CAD build for the part. Positions are in the model's coordinates, mm. A direction names the side the tool comes from. Round coordinates to 2 decimals unless told otherwise and drop trailing zeros. Loops run counter-clockwise (first coordinate to the right, second up) from the corner with the lowest first, then second, coordinate; pieces in that order, holes last. Notation, with made-up numbers: M 75,69 L 79,69 A15 ccw 79,92 Z; hole C 30.25,26 d2. An arc over 180 degrees is marked long. Use one line per item in the form item = value.
from build123d import *

# Parameters (mm, degrees)
SKETCH3_R           = 26.5
BOSS_EXTRUDE1_DEPTH = 37
SKETCH4_OUTSIDE_W   = 71.718
SKETCH4_OUTSIDE_H   = 71.718
SKETCH4_OUTSIDE_R   = 18.5
CUT_EXTRUDE1_DEPTH  = 1
SKETCH5_R           = 7.5
CUT_EXTRUDE2_DEPTH  = 2
CUT_EXTRUDE3_START  = -24.5
SKETCH6_W           = 30
SKETCH6_H           = 10
CUT_EXTRUDE3_DEPTH  = 29.16402947
CIRPATTERN1_COUNT   = 3
CIRPATTERN2_COUNT   = 3
CIRPATTERN3_COUNT   = 6


with BuildPart() as part:
    # Sketch3 → Boss-Extrude1 (new body)
    with BuildSketch(Plane.XY):
        Circle(SKETCH3_R)
    extrude(amount=-BOSS_EXTRUDE1_DEPTH)

    # Sketch4 outside → Cut-Extrude1 (cut)
    with BuildSketch(Plane.XY):
        Rectangle(SKETCH4_OUTSIDE_W, SKETCH4_OUTSIDE_H)
        Circle(SKETCH4_OUTSIDE_R, mode=Mode.SUBTRACT)
    extrude(amount=-CUT_EXTRUDE1_DEPTH, mode=Mode.SUBTRACT)

    # Sketch5 → Cut-Extrude2 (cut)
    with BuildSketch(Plane.XY):
        Circle(SKETCH5_R)
    extrude(amount=-CUT_EXTRUDE2_DEPTH, mode=Mode.SUBTRACT)

    # Sketch6 → Cut-Extrude3 (cut, through all)
    with BuildSketch(Plane.XY.offset(CUT_EXTRUDE3_START)):
        with Locations((0, -28)):
            Rectangle(SKETCH6_W, SKETCH6_H)
    extrude(amount=-CUT_EXTRUDE3_DEPTH, mode=Mode.SUBTRACT)

    # Sketch8 → M2.5x0.45 Tapped Hole1 (revolve, cut)
    with BuildSketch(Plane(origin=(-5.878275914, -23.011048917, -1), x_dir=(0, -1, 0), z_dir=(1, 0, 0))):
        Polygon((0, 0), (0, 6.965882135), (1.025, 6.35), (1.025, 0), align=None)
    m2_5x0_45_tapped_hole1 = revolve(axis=Axis((-5.878275914, -23.011048917, 5.35), (0, 0, -1)), mode=Mode.SUBTRACT)

    # Sketch10 → M2.5x0.45 Tapped Hole2 (revolve, cut)
    with BuildSketch(Plane(origin=(4.059528293, 12.875178835, 0), x_dir=(0, -1, 0), z_dir=(1, 0, 0))):
        Polygon((0, 0), (0, 4.965882135), (1.025, 4.35), (1.025, 0), align=None)
    m2_5x0_45_tapped_hole2 = revolve(axis=Axis((4.059528293, 12.875178835, 6.35), (0, 0, -1)), mode=Mode.SUBTRACT)

    # Sketch12 → M2.5x0.45 Tapped Hole3 (revolve, cut)
    with BuildSketch(Plane(origin=(0, 22.5, -37), x_dir=(0, 1, 0), z_dir=(1, 0, 0))):
        Polygon((0, 0), (0, 6.965882135), (1.025, 6.35), (1.025, 0), align=None)
    m2_5x0_45_tapped_hole3 = revolve(axis=Axis((0, 22.5, -43.35), (0, 0, 1)), mode=Mode.SUBTRACT)

    # CirPattern1: M2.5x0.45 Tapped Hole1 ×3 about axis
    cirpattern1_axis = Axis((0, 0, 0), (0, 0, 1))
    for i in range(1, CIRPATTERN1_COUNT):
        add(m2_5x0_45_tapped_hole1.rotate(cirpattern1_axis, i * 360 / CIRPATTERN1_COUNT), mode=Mode.SUBTRACT)

    # CirPattern2: M2.5x0.45 Tapped Hole2 ×3 about axis
    cirpattern2_axis = Axis((0, 0, 0), (0, 0, 1))
    for i in range(1, CIRPATTERN2_COUNT):
        add(m2_5x0_45_tapped_hole2.rotate(cirpattern2_axis, i * 360 / CIRPATTERN2_COUNT), mode=Mode.SUBTRACT)

    # CirPattern3: M2.5x0.45 Tapped Hole3 ×6 about axis, 1 skipped
    cirpattern3_axis = Axis((0, 0, 0), (0, 0, -1))
    add([m2_5x0_45_tapped_hole3.rotate(cirpattern3_axis, i * 360 / CIRPATTERN3_COUNT) for i in range(1, CIRPATTERN3_COUNT) if i not in (3,)], mode=Mode.SUBTRACT)


solid = part.part
1. Cut at D-D on z = -25.5. Write the cut outline in (x, y), and give its area (3 significant figures).
Completed:
outline = M -13.16,-23 L 13.16,-23 A26.5 ccw long Z
area = 2,140 mm2
2. Cut at A-A on y = 0. Write the cut outline in (x, z).
Completed:
outline = M -26.5,-37 L 26.5,-37 L 26.5,-1 L 18.5,-1 L 18.5,0 L 7.5,0 L 7.5,-2 L -7.5,-2 L -7.5,0 L -18.5,0 L -18.5,-1 L -26.5,-1 Z
3. Cut at C-C on x = -9. Write the cut outline in (y, z), and give its area (3 significant figures).
Completed:
outline = M -24.92,-24.5 L -23,-24.5 L -23,-37 L 24.92,-37 L 24.92,-1 L 16.16,-1 L 16.16,0 L -16.16,0 L -16.16,-1 L -24.92,-1 Z
area = 1,800 mm2
4. Cut at B-B on z = -3.5. Write the cut outline in (x, y) (3 decimals).
Completed:
outline = C 0,0 d53; hole C -16.989,16.596 d2.05; hole C -13.18,-2.922 d2.05; hole C -5.878,-23.011 d2.05; hole C 4.06,12.875 d2.05; hole C 9.12,-9.953 d2.05; hole C 22.867,6.415 d2.05
5. Pull direction Y, two halves, no side cores. Call faces 1 (the face through (0, 2, -37)), 2 (the face through (-3.45, 26.274, -18.748)), 3 (the face through (-0.045, 21.476, -33.869)): +Y half, -Y half, draft (parallel to the pull), parting line (faces both ways), or undercut.
Completed:
face_1 = draft
face_2 = parting line
face_3 = undercut
6. Tool access for faces 4 (the face through (-20.395, 10.777, -33.869)), 5 (the face through (0, 0, -2)), 6 (the face through (0, -24, -24.5)): list every direction of +Z, -Z, +X, -X, +Y, -Y with a clear straight run to the whole face (end or side of a thin tool).
Completed:
face_4 = -Z
face_5 = +Z
face_6 = -Z, +X, -X, -Y
7. Probe line 1 along Z through (x, y) = (-20, 15.5); line 2 along Y through (x, z) = (0.5, -18.5); line 3 along X through (y, z) = (-11, -34). List the from-to ranges inside material, lowest first. Write a range as from..to.
Completed:
line_1 = -37..-1
line_2 = -26.5..26.5
line_3 = -24.11..-20.48, -18.49..18.49, 20.48..24.11
8. Drop flat-ended pins along their axis: P1, Ø3, axis at y = 10, z = -22, coming from the +X side; P2, Ø6, axis at x = -4, z = -30, coming from the -Y side; P3, Ø3.5, axis at x = 0, y = 22.5, coming from the +Z side. Give the stop position or say it passes through.
Completed:
P1 = 25.1
P2 = -23
P3 = -1
